Can you work these out from the model? Positions are in its coordinate system, mm. A direction names the side the tool comes from. Round coordinates to 2 decimals unless told otherwise and drop trailing zeros. Loops run counter-clockwise (first coordinate to the right, second up) from the corner with the lowest first, then second, coordinate; pieces in that order, holes last. Notation, with made-up numbers: (58, -36) -> (117, -36) arc R37 cw to (117, 3) -> close; hole circle Ø10 at (-8.5, 10). An arc over 180 degrees is marked (long way). Use a Markdown table: item, result.
from build123d import *

# Parameters (mm, degrees)
BOSS_EXTRUDE1_DEPTH      = 25
BOSS_EXTRUDE1_DEPTH_BACK = 25
SKETCH2_W                = 74.2
SKETCH2_H                = 66.1
CUT_EXTRUDE1_DEPTH       = 25
CUT_EXTRUDE1_DEPTH_BACK  = 25
SKETCH3_R                = 3
CUT_EXTRUDE2_DEPTH       = 12.1
CUT_EXTRUDE2_DEPTH_BACK  = 12.1
SKETCH4_R                = 2.75
CUT_EXTRUDE3_DEPTH       = 3
CUT_EXTRUDE3_DEPTH_BACK  = 3
SKETCH5_R                = 2.75
CUT_EXTRUDE4_DEPTH       = 3
CUT_EXTRUDE4_DEPTH_BACK  = 3


with BuildPart() as part:
    # Sketch1 → Boss-Extrude1 (new body, two sides)
    with BuildSketch(Plane(origin=(0, 0, 0), x_dir=(0, 0, -1), z_dir=(1, 0, 0))) as boss_extrude1_sk:
        with BuildLine():
            Line((-6.05, 0), (6.05, 0))
            ThreePointArc((6.05, 0), (8.171320344, 0.878679656), (9.05, 3))
            Line((9.05, 3), (9.05, 34))
            Line((9.05, 34), (6.05, 34))
            Line((6.05, 34), (6.05, 4.6))
            ThreePointArc((6.05, 4.6), (5.58137085, 3.46862915), (4.45, 3))
            Line((4.45, 3), (-4.45, 3))
            ThreePointArc((-4.45, 3), (-5.58137085, 3.46862915), (-6.05, 4.6))
            Line((-6.05, 4.6), (-6.05, 34))
            Line((-6.05, 34), (-9.05, 34))
            Line((-9.05, 34), (-9.05, 3))
            ThreePointArc((-9.05, 3), (-8.171320344, 0.878679656), (-6.05, 0))
        make_face()
    extrude(amount=BOSS_EXTRUDE1_DEPTH)
    extrude(boss_extrude1_sk.sketch, amount=-BOSS_EXTRUDE1_DEPTH_BACK)

    # Sketch2 → Cut-Extrude1 (cut, two sides)
    with BuildSketch(Plane.XY) as cut_extrude1_sk:
        with Locations((0, 20.95)):
            Rectangle(SKETCH2_W, SKETCH2_H)
        with BuildLine():
            Line((0, 0), (25, 0))
            Line((25, 0), (25, 3))
            Line((25, 3), (13.425422134, 29.777399934))
            ThreePointArc((13.425422134, 29.777399934), (5.58189474, 33.854850653), (0, 27))
            Line((0, 27), (0, 0))
        make_face(mode=Mode.SUBTRACT)
    extrude(amount=CUT_EXTRUDE1_DEPTH, mode=Mode.SUBTRACT)
    extrude(cut_extrude1_sk.sketch, amount=-CUT_EXTRUDE1_DEPTH_BACK, mode=Mode.SUBTRACT)

    # Sketch3 → Cut-Extrude2 (cut, two sides)
    with BuildSketch(Plane.XY) as cut_extrude2_sk:
        with Locations((7, 27)):
            Circle(SKETCH3_R)
    extrude(amount=CUT_EXTRUDE2_DEPTH, mode=Mode.SUBTRACT)
    extrude(cut_extrude2_sk.sketch, amount=-CUT_EXTRUDE2_DEPTH_BACK, mode=Mode.SUBTRACT)

    # Sketch4 → Cut-Extrude3 (cut, two sides)
    with BuildSketch(Plane(origin=(0, 0, 0), x_dir=(1, 0, 0), z_dir=(0, 1, 0))) as cut_extrude3_sk:
        with Locations((5, 0)):
            Circle(SKETCH4_R)
    extrude(amount=CUT_EXTRUDE3_DEPTH, mode=Mode.SUBTRACT)
    extrude(cut_extrude3_sk.sketch, amount=-CUT_EXTRUDE3_DEPTH_BACK, mode=Mode.SUBTRACT)

    # Sketch5 → Cut-Extrude4 (cut, two sides)
    with BuildSketch(Plane(origin=(0, 0, 0), x_dir=(1, 0, 0), z_dir=(0, 1, 0))) as cut_extrude4_sk:
        with Locations((20, 0)):
            Circle(SKETCH5_R)
    extrude(amount=CUT_EXTRUDE4_DEPTH, mode=Mode.SUBTRACT)
    extrude(cut_extrude4_sk.sketch, amount=-CUT_EXTRUDE4_DEPTH_BACK, mode=Mode.SUBTRACT)


solid = part.part
1. I want a section at B-B (y = 25.5). Please give me the cut outline in (x, z).
Answer sheet:
| item | result |
|---|---|
| outline | (0, -9.05) -> (4.4, -9.05) -> (4.4, -6.05) -> (0, -6.05) -> close; (0, 6.05) -> (4.4, 6.05) -> (4.4, 9.05) -> (0, 9.05) -> close; (9.6, -9.05) -> (15.27, -9.05) -> (15.27, -6.05) -> (9.6, -6.05) -> close; (9.6, 6.05) -> (15.27, 6.05) -> (15.27, 9.05) -> (9.6, 9.05) -> close |
2. Will these pins go through, and if not, where does the flat tip stop? pin 1 Ø9 at (x, z) = (20, 0) entering from -Y; pin 2 Ø4.5 at (x, z) = (9.5, -2) entering from +Y; pin 3 Ø3 at (x, z) = (3, -4) entering from +Y.
Answer sheet:
| item | result |
|---|---|
| pin 1 | stops at y = 0 |
| pin 2 | stops at y = 3 |
| pin 3 | stops at y = 3.39 |
3. I want a section at A-A (z = 0). Please give me the cut outline in (x, y), plus the area to 3 significant figures.
Answer sheet:
| item | result |
|---|---|
| outline | (0, 0) -> (2.25, 0) -> (2.25, 3) -> (0, 3) -> close; (7.75, 0) -> (17.25, 0) -> (17.25, 3) -> (7.75, 3) -> close; (22.75, 0) -> (25, 0) -> (25, 3) -> (22.75, 3) -> close |
| area | 42.0 mm² |
4. I need wall thicknesses on line 1 (X direction, y = 1, z = 0); line 2 (Z direction, x = 15, y = 20); line 3 (Y direction, x = 17, z = -2.5). Which ranges of each line are inside material? Lowest first, please.
Answer sheet:
| item | result |
|---|---|
| line 1 | x = 0 to 2.25, 7.75 to 17.25, 22.75 to 25 |
| line 2 | z = -9.05 to -6.05, 6.05 to 9.05 |
| line 3 | y = 0 to 3 |
5. Which directions (+Z, -Z, +X, -X, +Y, -Y) give clear straight access to the entire face, cutting with the end or side of a thin tool? Please do faces 4 (the flat face through (13, 0, 0)), 5 (the cylindrical face through (12.68, 3.46, 5.57)).
Answer sheet:
| item | result |
|---|---|
| face 4 | +Z, -Z, +X, -X, -Y |
| face 5 | +X, -X, +Y |
6. I want a section at D-D (y = 19). Please give me the cut outline in (x, z), plus the area to 3 significant figures.
Answer sheet:
| item | result |
|---|---|
| outline | (0, -9.05) -> (18.08, -9.05) -> (18.08, -6.05) -> (0, -6.05) -> close; (0, 6.05) -> (18.08, 6.05) -> (18.08, 9.05) -> (0, 9.05) -> close |
| area | 109 mm² |
7. If we mould it in two halves opening along X, with no side actions, what happens to faces 1 (the flat face through (19.294, 16.201, 7.229)), 2 (the flat face through (10, 16, 6.05)), 3 (the cylindrical face through (7.54, 1.48, 1.05))? For each: +X half, -X half, draft (parallel to the pull), parting line (faces both ways), or undercut.
Answer sheet:
| item | result |
|---|---|
| face 1 | +X half |
| face 2 | draft |
| face 3 | undercut |
8. I want a section at C-C (x = 8.5). Please give me the cut outline in (y, z), plus the area to 3 significant figures.
Answer sheet:
| item | result |
|---|---|
| outline | (0, -6.05) arc R3 ccw to (3, -9.05) -> (24.4, -9.05) -> (24.4, -6.05) -> (4.6, -6.05) arc R1.6 cw to (3, -4.45) -> (3, 4.45) arc R1.6 cw to (4.6, 6.05) -> (24.4, 6.05) -> (24.4, 9.05) -> (3, 9.05) arc R3 ccw to (0, 6.05) -> close; (29.6, -9.05) -> (33.84, -9.05) -> (33.84, -6.05) -> (29.6, -6.05) -> close; (29.6, 6.05) -> (33.84, 6.05) -> (33.84, 9.05) -> (29.6, 9.05) -> close |
| area | 205 mm² |
